Design review of the part shown in the three views and the two pictorial views. Dimensions are in mm from the part's minimum x, y and z. A direction names the side the tool comes from. Coordinates: 2 decimals unless noted, no trailing zeros. Write each loop counter-clockwise with the first axis right and the second up, starting at its lowest first coordinate (ties: lowest second). Pieces come first, ordered by that corner, then holes. Notation, with made-up numbers: (31.5, 75) -> (43.5, 75) arc R17 ccw to (43.5, 86) -> close; hole circle Ø9 at (6.25, 58). An arc over 180 degrees is marked (long way). Write item = value, one per line. Start each with the question number.
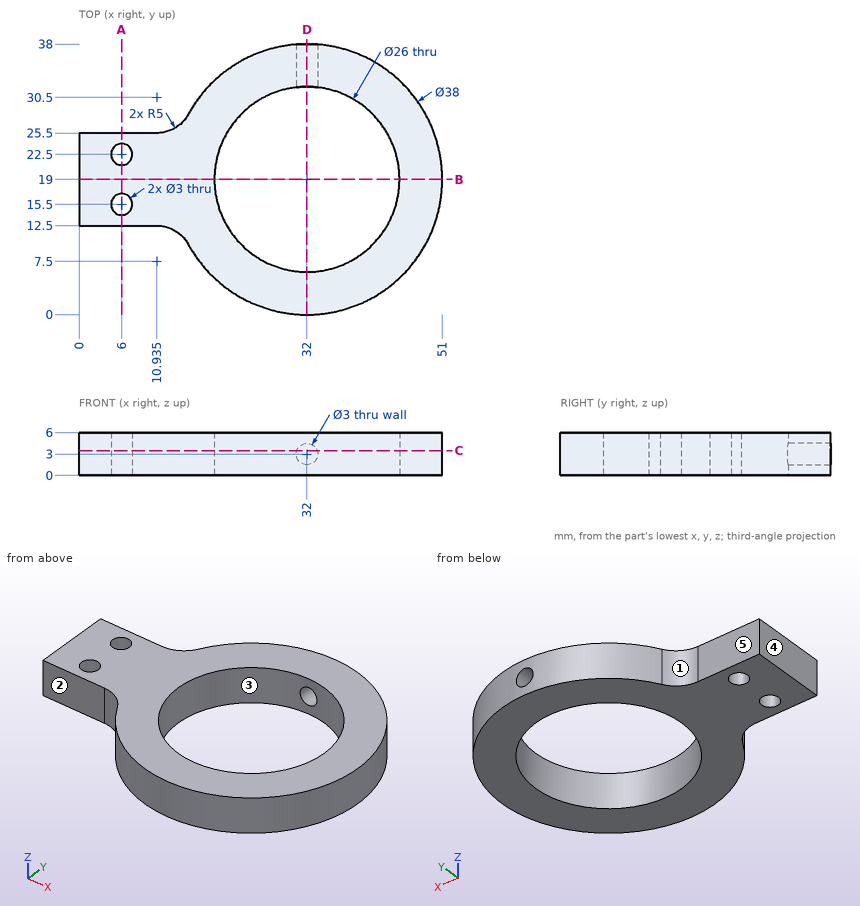
(1) For pin 1 Ø2 at (y, z) = (21.5, 5) entering from +X; pin 2 Ø1.8 at (x, z) = (4.5, 1.5) entering from +Y; pin 3 Ø1 at (x, z) = (42, 2) entering from -Y (1 decimal), all flat-tipped, find the tip position at first contact; note any pin that passes through.
(2) For the marked faces 4 and 5, list the 3-axis set-ups (+Z, -Z, +X, -X, +Y, -Y) from which the entire face can be reached by the end or side of a thin tool; tool diameter is ignored.
(3) Take a section at D-D, the plane x = 32. State the section outline as (y, z) points.
(4) For line 1 (Y direction, x = 6, z = 1.2); line 2 (Z direction, x = 32, y = 33); line 3 (X direction, y = 23.5, z = 2.5) (1 decimal), list the stretches that pass through material, from the lowest coordinate up.
(5) Take a section at A-A, the plane x = 6. State the section outline as (y, z) points.
(6) Take a section at C-C, the plane z = 3.5. State the section outline as (x, y) points (1 decimal).
(7) Take a section at B-B, the plane y = 19. State the section outline as (x, z) points.
(8) Mouldability with a two-part tool opening along Y and no side actions: class the marked faces 1, 2 and 3 as pulls with the +Y half, pulls with the -Y half, needs draft (parallel to the pull), parting line crosses it, or undercut.
Report:
q1.pin_1 = 50.94
q1.pin_2 = 25.5
q1.pin_3 = 2.5
q2.face_4 = +Z, -Z, -X, +Y, -Y
q2.face_5 = +Z, -Z, -X, +Y
q3.outline = (0, 0) -> (6, 0) -> (6, 6) -> (0, 6) -> close; (32, 0) -> (38, 0) -> (38, 1.5) -> (32, 1.5) -> close; (32, 4.5) -> (38, 4.5) -> (38, 6) -> (32, 6) -> close
q4.line_1 = 12.5 to 14, 17 to 21, 24 to 25.5
q4.line_2 = 0 to 1.5, 4.5 to 6
q4.line_3 = 0 to 4.9, 7.1 to 19.8, 44.2 to 50.5
q5.outline = (12.5, 0) -> (14, 0) -> (14, 6) -> (12.5, 6) -> close; (17, 0) -> (21, 0) -> (21, 6) -> (17, 6) -> close; (24, 0) -> (25.5, 0) -> (25.5, 6) -> (24, 6) -> close
q6.outline = (0, 12.5) -> (10.9, 12.5) arc R5 cw to (15.3, 9.9) arc R19 ccw (long way) to (33.4, 37.9) -> (33.4, 31.9) arc R13 cw (long way) to (30.6, 31.9) -> (30.6, 37.9) arc R19 ccw to (15.3, 28.1) arc R5 cw to (10.9, 25.5) -> (0, 25.5) -> close; hole circle Ø3 at (6, 15.5); hole circle Ø3 at (6, 22.5)
q7.outline = (0, 0) -> (19, 0) -> (19, 6) -> (0, 6) -> close; (45, 0) -> (51, 0) -> (51, 6) -> (45, 6) -> close
q8.face_1 = pulls with the +Y half
q8.face_2 = pulls with the -Y half
q8.face_3 = undercut
